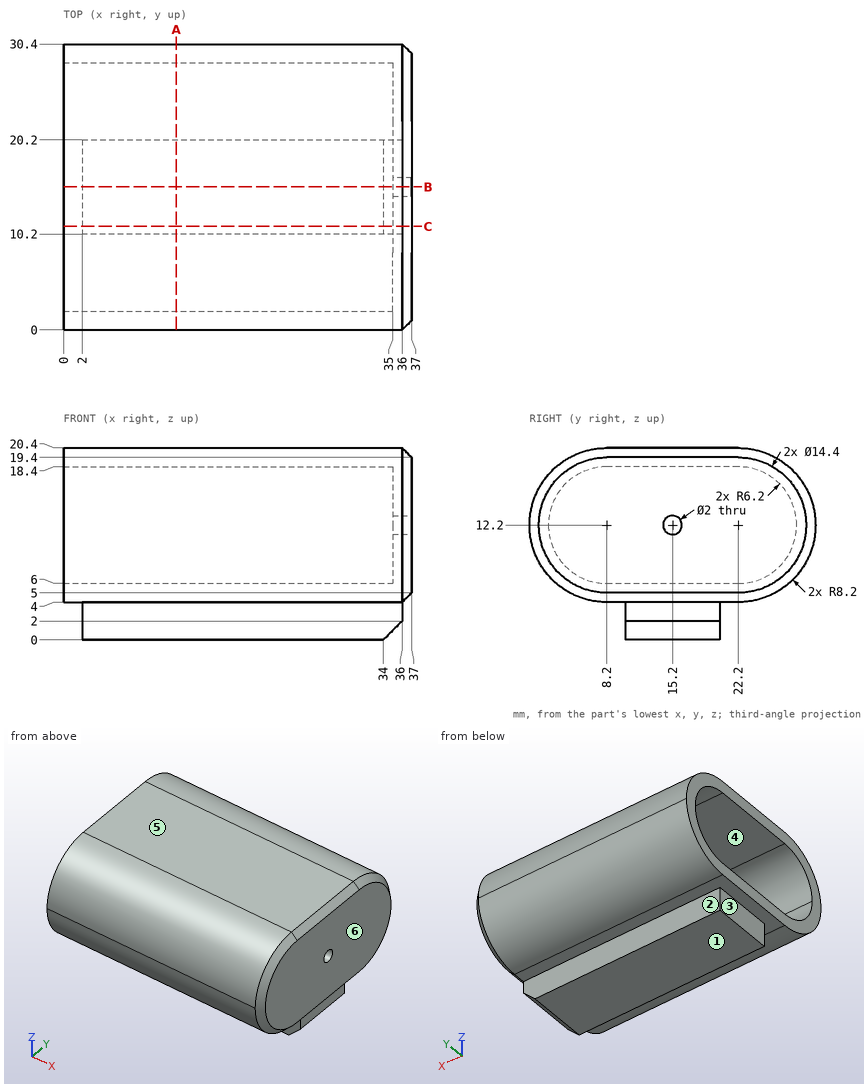
Print and shaded views of the part. All mm, measured from the part's lowest x, y and z. A direction names the side the tool comes from. Give positions to 0.01 mm unless a question says otherwise; leave off trailing zeros. Order: outer loops, then holes, each group sorted by start corner. A loop starts at its lowest first (then second) coordinate and runs counter-clockwise, first axis right, second up. Notation, with made-up numbers: (18.5, 19.5) - (57.5, 19.5) arc R19 ccw to (57.5, 41.5) - close; hole circle Ø10 at (-14, -4.75). An arc over 180 degrees is marked (long way). One line per item, written item: value.
Item 1: Slice it at A-A (x = 12). List the corners of the cut face in (y, z), then the cut area to 3 significant figures.
Response values:
outline: (8.2, 4) - (10.2, 4) - (10.2, 0) - (20.2, 0) - (20.2, 4) - (22.2, 4) arc R8.2 ccw to (22.2, 20.4) - (8.2, 20.4) arc R8.2 ccw to start; hole (8.2, 6) - (22.2, 6) arc R6.2 ccw to (22.2, 18.4) - (8.2, 18.4) arc R6.2 ccw to start
area: 186 mm2
Item 2: Slice it at C-C (y = 11). List the corners of the cut face in (x, z).
Response values:
outline: (0, 4) - (2, 4) - (2, 0) - (34, 0) - (36, 2) - (36, 4) - (37, 5) - (37, 19.4) - (36, 20.4) - (0, 20.4) - (0, 18.4) - (35, 18.4) - (35, 6) - (0, 6) - close
Item 3: Slice it at B-B (y = 15.2). List the corners of the cut face in (x, z), then the cut area to 3 significant figures.
Response values:
outline: (0, 4) - (2, 4) - (2, 0) - (34, 0) - (36, 2) - (36, 4) - (37, 5) - (37, 11.2) - (35, 11.2) - (35, 6) - (0, 6) - close; (0, 18.4) - (35, 18.4) - (35, 13.2) - (37, 13.2) - (37, 19.4) - (36, 20.4) - (0, 20.4) - close
area: 302 mm2
Item 4: Wall check: line 1 (Z direction, x = 18.5, y = 12.5); line 2 (Y direction, x = 31, z = 1.75); line 3 (Z direction, x = 20, y = 22). Give the ranges that are in metal, low to high.
Response values:
line 1: 0 to 6, 18.4 to 20.4
line 2: 10.2 to 20.2
line 3: 4 to 6, 18.4 to 20.4
Item 5: Pin check, flat tips, straight feed: pin 1 Ø5 at (x, y) = (18, 4) entering from +Z; pin 2 Ø4 at (x, z) = (28.5, 5) entering from -Y; pin 3 Ø1.6 at (y, z) = (15.2, 12.2) entering from +X; pin 4 Ø3 at (x, z) = (24.5, 17) entering from +Y. Stop position of each tip, or through.
Response values:
pin 1: z = 20.22
pin 2: y = 1.86
pin 3: through
pin 4: y = 29.71
Item 6: Two-plate mould, pull along Z, no slides. Class the marked faces 4, 5 and 6: released by +Z, released by -Z, zero draft, split by the parting line, or undercut.
Response values:
face 4: undercut
face 5: released by +Z
face 6: zero draft
Item 7: Tool access for the marked faces 1, 2 and 3: list every direction of +Z, -Z, +X, -X, +Y, -Y with a clear straight run to the whole face (end or side of a thin tool).
Response values:
face 1: -Z, +X, -X, +Y, -Y
face 2: -Z, +X, -X, +Y
face 3: -Z, -X, +Y, -Y
